Autodesk Inventor part; units mm, degrees
ref_plane "YZ Plane" through (0, 0, 0) normal (1, 0, 0) x (0, 1, 0)
ref_plane "XZ Plane" through (0, 0, 0) normal (0, 1, 0) x (-1, 0, 0)
ref_plane "XY Plane" through (0, 0, 0) normal (0, 0, 1) x (1, 0, 0)
sketch "スケッチ1" plane through (0, 0, 0) normal (0, 0, 1) x (1, 0, 0)
  line L0 (0, 0) -> (30, 0)
  line L1 (30, 0) -> (30, 20)
  line L2 (30, 20) -> (0, 20)
  line L3 (0, 20) -> (0, 0)
  dimension "d0" = 20
  dimension "d1" = 30
extrude "押し出し1" add sketch "スケッチ1" along normal blind 1
sketch "スケッチ2" plane through (0, 0, 1) normal (0, 0, 1) x (1, 0, 0)
  line L0 (30, 20) -> (0, 20)
  point P0 (0, 0)
  point P1 (15, 12)
  point P2 (15, 20)
  dimension "d4" = 8
hole "穴1" at (15, 12, 1) direction (0, 0, -1) diameter 4.5 end through all
sketch "スケッチ3" plane through (0, 0, 1) normal (0, 0, 1) x (1, 0, 0)
  line L0 (0, 20) -> (0, 0)
  line L1 (0, 0) -> (30, 0)
  line L2 (30, 20) -> (0, 20)
  point P0 (4, 5.25)
  point P1 (26, 5.25)
  dimension "d12" = 22
  dimension "d13" = 4
  dimension "d22" = 14.75
hole "穴2" at (4, 5.25, 1) at (26, 5.25, 1) direction (0, 0, -1) diameter 3.2 end through all
properties part number "CLS_typeC_31.4N_plate"
Geometry check sheet. Reference: the model listing, model coordinates, mm. Round coordinates to 2 decimals unless told otherwise and drop trailing zeros. Loops run counter-clockwise (first coordinate to the right, second up) from the corner with the lowest first, then second, coordinate; pieces in that order, holes last. Notation, with made-up numbers: (72, -30.5) -> (83, -30.5) arc R28 ccw to (83, -9.5) -> close; hole circle Ø3 at (34.25, 67). An arc over 180 degrees is marked (long way). Use a Markdown table: item, result.
(1) Sectioned sample at D-D (y = 5.25). Enter the section's corners in (x, z).
Calculated:
| item | result |
|---|---|
| outline | (0, 0) -> (2.4, 0) -> (2.4, 1) -> (0, 1) -> close; (5.6, 0) -> (24.4, 0) -> (24.4, 1) -> (5.6, 1) -> close; (27.6, 0) -> (30, 0) -> (30, 1) -> (27.6, 1) -> close |
(2) Mould release check, pull along Y, two halves, no side actions. Record for faces 1 (the flat face through (0, 10.1, 0.5)), 2 (the flat face through (15.2, 20, 0.5)), 3 (the cylindrical face through (24.414, 5.458, 0.493)): released by +Y, released by -Y, zero draft, split by the parting line, or undercut.
Calculated:
| item | result |
|---|---|
| face 1 | zero draft |
| face 2 | released by +Y |
| face 3 | undercut |
(3) Sectioned sample at C-C (z = 0.3). Enter the section's corners in (x, y), then the cut area to 3 significant figures.
Calculated:
| item | result |
|---|---|
| outline | (0, 0) -> (30, 0) -> (30, 20) -> (0, 20) -> close; hole circle Ø3.2 at (4, 5.25); hole circle Ø4.5 at (15, 12); hole circle Ø3.2 at (26, 5.25) |
| area | 568 mm² |
(4) Sectioned sample at A-A (x = 26). Enter the section's corners in (y, z).
Calculated:
| item | result |
|---|---|
| outline | (0, 0) -> (3.65, 0) -> (3.65, 1) -> (0, 1) -> close; (6.85, 0) -> (20, 0) -> (20, 1) -> (6.85, 1) -> close |
(5) Scan lines: probe 1 along X at (y, z) = (5.25, 0.6); probe 2 along Y at (x, z) = (26, 0.4); probe 3 along X at (y, z) = (12, 0.3). Record each from-to range of solid material in increasing order.
Calculated:
| item | result |
|---|---|
| probe 1 | 0 to 2.4, 5.6 to 24.4, 27.6 to 30 |
| probe 2 | 0 to 3.65, 6.85 to 20 |
| probe 3 | 0 to 12.75, 17.25 to 30 |
(6) Sectioned sample at B-B (y = 12). Enter the section's corners in (x, z), then the cut area to 3 significant figures.
Calculated:
| item | result |
|---|---|
| outline | (0, 0) -> (12.75, 0) -> (12.75, 1) -> (0, 1) -> close; (17.25, 0) -> (30, 0) -> (30, 1) -> (17.25, 1) -> close |
| area | 25.5 mm² |
